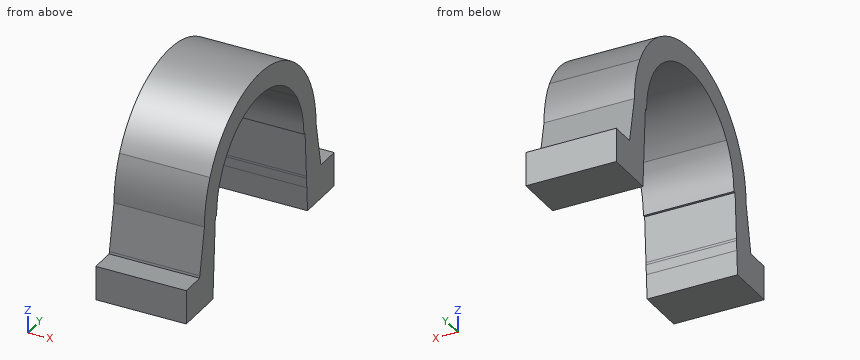
from build123d import *

# Parameters (mm, degrees)
F1_DEPTH = 20


with BuildPart() as f1:
    # F0 (on Right) → F1 (new body)
    with BuildSketch(Plane.YZ):
        with BuildLine():
            ThreePointArc((14.9666295471, 10), (17.2249721603, 5.2249721603), (18, 0))
            Line((18, 0), (18.5, 0))
            Line((18.5, 0), (23, 0))
            ThreePointArc((23, 0), (22.4207855469, 5.1291690811), (20.7123151772, 10))
            Line((20.7123151772, 10), (14.9666295471, 10))
        make_face()
        with BuildLine():
            ThreePointArc((-14.9666295471, 10), (0, 18), (14.9666295471, 10))
            Line((14.9666295471, 10), (20.7123151772, 10))
            ThreePointArc((20.7123151772, 10), (0, 23), (-20.7123151772, 10))
            Line((-20.7123151772, 10), (-14.9666295471, 10))
        make_face()
        with BuildLine():
            Line((23, 0), (18.5, 0))
            Line((18.5, 0), (19.0555555556, -10))
            Line((19.0555555556, -10), (20.7123151772, -10))
            ThreePointArc((20.7123151772, -10), (22.4207855469, -5.1291690811), (23, 0))
        make_face()
        with BuildLine():
            ThreePointArc((-18, 0), (-17.2249721603, 5.2249721603), (-14.9666295471, 10))
            Line((-14.9666295471, 10), (-20.7123151772, 10))
            ThreePointArc((-20.7123151772, 10), (-22.4207855469, 5.1291690811), (-23, 0))
            Line((-23, 0), (-18.5, 0))
            Line((-18.5, 0), (-18, 0))
        make_face()
        with BuildLine():
            Line((23, -10), (23, 0))
            ThreePointArc((23, 0), (22.4207855469, -5.1291690811), (20.7123151772, -10))
            Line((20.7123151772, -10), (23, -10))
        make_face()
        Polygon((24.9047619048, -10), (23, 0), (23, -10), align=None)
        with BuildLine():
            Line((20.7123151772, -10), (19.0555555556, -10))
            Line((19.0555555556, -10), (19.0833333333, -10.5))
            Line((19.0833333333, -10.5), (20.4633819297, -10.5))
            ThreePointArc((20.4633819297, -10.5), (20.5893663831, -10.2507556766), (20.7123151772, -10))
        make_face()
        with BuildLine():
            Line((-19.0555555556, -10), (-18.5, 0))
            Line((-18.5, 0), (-23, 0))
            ThreePointArc((-23, 0), (-22.4207855469, -5.1291690811), (-20.7123151772, -10))
            Line((-20.7123151772, -10), (-19.0555555556, -10))
        make_face()
        with BuildLine():
            Line((23, -10), (20.7123151772, -10))
            ThreePointArc((20.7123151772, -10), (20.5893663831, -10.2507556766), (20.4633819297, -10.5))
            Line((20.4633819297, -10.5), (23, -10.5))
            Line((23, -10.5), (23, -10))
        make_face()
        Polygon((24.9047619048, -10), (23, -10), (23, -10.5), (25, -10.5), align=None)
        with BuildLine():
            Line((20.4633819297, -10.5), (19.0833333333, -10.5))
            Line((19.0833333333, -10.5), (19.2032450764, -12.6584113749))
            ThreePointArc((19.2032450764, -12.6584113749), (19.862653635, -11.5963352217), (20.4633819297, -10.5))
        make_face()
        with BuildLine():
            ThreePointArc((-20.7123151772, -10), (-22.4207855469, -5.1291690811), (-23, 0))
            Line((-23, 0), (-24.9047619048, -10))
            Line((-24.9047619048, -10), (-20.7123151772, -10))
        make_face()
        with BuildLine():
            Line((-19.0833333333, -10.5), (-19.0555555556, -10))
            Line((-19.0555555556, -10), (-20.7123151772, -10))
            ThreePointArc((-20.7123151772, -10), (-20.5893663831, -10.2507556766), (-20.4633819297, -10.5))
            Line((-20.4633819297, -10.5), (-19.0833333333, -10.5))
        make_face()
        with BuildLine():
            Line((-19.5, -18), (-19.2032450764, -12.6584113749))
            ThreePointArc((-19.2032450764, -12.6584113749), (-19.862653635, -11.5963352217), (-20.4633819297, -10.5))
            Line((-20.4633819297, -10.5), (-25, -10.5))
            Line((-25, -10.5), (-30.5, -10.5))
            Line((-30.5, -10.5), (-30.5, -18))
            Line((-30.5, -18), (-19.5, -18))
        make_face()
        with BuildLine():
            ThreePointArc((-20.4633819297, -10.5), (-19.862653635, -11.5963352217), (-19.2032450764, -12.6584113749))
            Line((-19.2032450764, -12.6584113749), (-19.0833333333, -10.5))
            Line((-19.0833333333, -10.5), (-20.4633819297, -10.5))
        make_face()
        with BuildLine():
            Line((23, -10.5), (20.4633819297, -10.5))
            ThreePointArc((20.4633819297, -10.5), (19.862653635, -11.5963352217), (19.2032450764, -12.6584113749))
            Line((19.2032450764, -12.6584113749), (19.5, -18))
            Line((19.5, -18), (30.5, -18))
            Line((30.5, -18), (30.5, -10.5))
            Line((30.5, -10.5), (25, -10.5))
            Line((25, -10.5), (23, -10.5))
        make_face()
        with BuildLine():
            ThreePointArc((-20.4633819297, -10.5), (-20.5893663831, -10.2507556766), (-20.7123151772, -10))
            Line((-20.7123151772, -10), (-24.9047619048, -10))
            Line((-24.9047619048, -10), (-25, -10.5))
            Line((-25, -10.5), (-20.4633819297, -10.5))
        make_face()
    extrude(amount=F1_DEPTH)


solid = f1.part
Read the model definition and answer for the solid it produces. Units are mm, in the model's axes. Coordinates: 2 decimals unless noted, no trailing zeros. Order: outer loops, then holes, each group sorted by start corner. A loop starts at its lowest first (then second) coordinate and runs counter-clockwise, first axis right, second up. Notation, with made-up numbers: M -11,38 L 10,38 A10 ccw 10,47 Z; hole C 66,-18.75 d6. An arc over 180 degrees is marked long. Put each result on its own line as item: value. Start each with the question number.
Item 1: Section B-B, the plane z = -6 is taken. Determine the outline of the cut face in (x, y), plus the area to 3 significant figures.
Item 2: Section C-C, the plane z = 15.5 is taken. Determine the outline of the cut face in (x, y).
Item 3: Consider probe 1 along Z at (x, y) = (10.75, -26.5); probe 2 along Y at (x, z) = (3.5, 15.5); probe 3 along Y at (x, z) = (11.5, 6). Determine where each line is inside the solid, lowest interval first. Write a range as [from, to].
Item 4: Section D-D, the plane y = -11 is taken. Determine the outline of the cut face in (x, z).
Item 5: Section A-A, the plane x = 18.5 is taken. Determine the outline of the cut face in (y, z).
Item 6: Given pin 1 Ø1.5 at (x, y) = (9, 9) entering from -Z; pin 2 Ø6 at (y, z) = (-2.5, 14.5) entering from -X; pin 3 Ø1 at (x, y) = (2.5, 4.5) entering from +Z; pin 4 Ø1 at (x, z) = (16.5, 16) entering from +Y, each flat-ended and moving along its own axis, determine where each tip first touches the part or whether it passes through.
Computed:
1. outline: M 0,-24.14 L 20,-24.14 L 20,-18.83 L 0,-18.83 Z; M 0,18.83 L 20,18.83 L 20,24.14 L 0,24.14 Z
1. area: 212 mm2
2. outline: M 0,-16.99 L 20,-16.99 L 20,-9.15 L 0,-9.15 Z; M 0,9.15 L 20,9.15 L 20,16.99 L 0,16.99 Z
3. probe 1: z = [-18, -10.5]
3. probe 2: y = [-16.99, -9.15], [9.15, 16.99]
3. probe 3: y = [-22.2, -16.97], [16.97, 22.2]
4. outline: M 0,14.25 L 20,14.25 L 20,20.2 L 0,20.2 Z
5. outline: M -30.5,-18 L -19.5,-18 L -18.5,0 L -18,0 A18 cw 18,0 L 18.5,0 L 19.5,-18 L 30.5,-18 L 30.5,-10.5 L 25,-10.5 L 23,0 A23 ccw -23,0 L -25,-10.5 L -30.5,-10.5 Z
6. pin 1: stops at z = 15.13
6. pin 2: passes through
6. pin 3: stops at z = 22.65
6. pin 4: stops at y = 16.99
